```python
from build123d import *

# Parameters (mm, degrees)
F1_DEPTH = 20.55
F2_W     = 14.525
F2_H     = 29.4
F2_W_2   = 29.4
F2_H_2   = 14.525
F3_DEPTH = 20.551
F4_W     = 29.4
F4_H     = 30
F4_W_2   = 30
F4_H_2   = 29.4
F5_DEPTH = 20.55


with BuildPart() as f1:
    # F0 (on Top) → F1 (new body)
    with BuildSketch(Plane.XY):
        Polygon((-60.225, 60.225), (89.625, 60.225), (89.625, 89.625), (-89.625, 89.625), (-89.625, -89.625), (-60.225, -89.625), align=None)
    extrude(amount=F1_DEPTH)

    # F2 (on face) → F3 (cut, through all)
    with BuildSketch(Plane.XY.offset(20.55)):
        with Locations((82.3625, 74.925)):
            Rectangle(F2_W, F2_H)
        with Locations((-74.925, -82.3625)):
            Rectangle(F2_W_2, F2_H_2)
    extrude(amount=-F3_DEPTH, mode=Mode.SUBTRACT)

    # F4 (on Top) → F5 (join, through all)
    with BuildSketch(Plane.XY):
        with Locations((-74.925, -90.1)):
            Rectangle(F4_W, F4_H)
        with Locations((90.1, 74.925)):
            Rectangle(F4_W_2, F4_H_2)
    extrude(amount=F5_DEPTH)


solid = f1.part
```
The model under review builds one solid part; all positions refer to its coordinate system, in mm. A direction names the side the tool comes from. Give positions to 0.01 mm unless a question says otherwise; leave off trailing zeros. Write each loop counter-clockwise with the first axis right and the second up, starting at its lowest first coordinate (ties: lowest second). Pieces come first, ordered by that corner, then holes.
(1) Consider section A-A, the plane x = -7.5. Give the boundary of the cut face in (y, z) (3 decimals), and give its area (3 significant figures).
(2) For P1, Ø6, axis at y = -14.5, z = 5.5, coming from the +X side (3 decimals); P2, Ø6, axis at x = -13, z = 6, coming from the -Y side (3 decimals), all flat-tipped, find the tip position at first contact; note any pin that passes through.
(3) To check wall thickness, follow L1, parallel to Y at x = 51, z = 2 (3 decimals); L2, parallel to X at y = 22.5, z = 16.75 (3 decimals). State the ranges of each line that lie inside material, in increasing order.
(4) Tool access review of faces 1 (the flat face through (-60.225, -24, 10)), 2 (the flat face through (-36, 65, 20.55)): name each direction out of +Z, -Z, +X, -X, +Y, -Y from which nothing blocks a thin tool from reaching the whole face with its end or side.
(5) Consider section C-C, the plane y = 23.5. Give the boundary of the cut face in (x, z) (3 decimals), and give its area (3 significant figures).
(6) Consider section B-B, the plane z = 4.25. Give the boundary of the cut face in (x, y) (3 decimals), and give its area (3 significant figures).
Returned:
1. outline: (60.225, 0) - (89.625, 0) - (89.625, 20.55) - (60.225, 20.55) - close
1. area: 604 mm2
2. P1: stops at x = -60.225
2. P2: stops at y = 60.225
3. L1: y = 60.225 to 89.625
3. L2: x = -89.625 to -60.225
4. face 1: +Z, -Z, +X, -Y
4. face 2: +Z, +X, -X, +Y, -Y
5. outline: (-89.625, 0) - (-60.225, 0) - (-60.225, 20.55) - (-89.625, 20.55) - close
5. area: 604 mm2
6. outline: (-89.625, -105.1) - (-60.225, -105.1) - (-60.225, 60.225) - (105.1, 60.225) - (105.1, 89.625) - (-89.625, 89.625) - close
6. area: 10,600 mm2
